Source: three-view drawing plus pictorial views. Frame: mm from the lowest corner of the part. A direction names the side the tool comes from. Give positions to 0.01 mm unless a question says otherwise; leave off trailing zeros. Loops run counter-clockwise (first coordinate to the right, second up) from the corner with the lowest first, then second, coordinate; pieces in that order, holes last. Notation, with made-up numbers: M 46.5,19 L 52.5,19 A18 ccw 52.5,47 Z; hole C 40,39.25 d10. An arc over 180 degrees is marked long. Put each result on its own line as item: value. Start each with the question number.
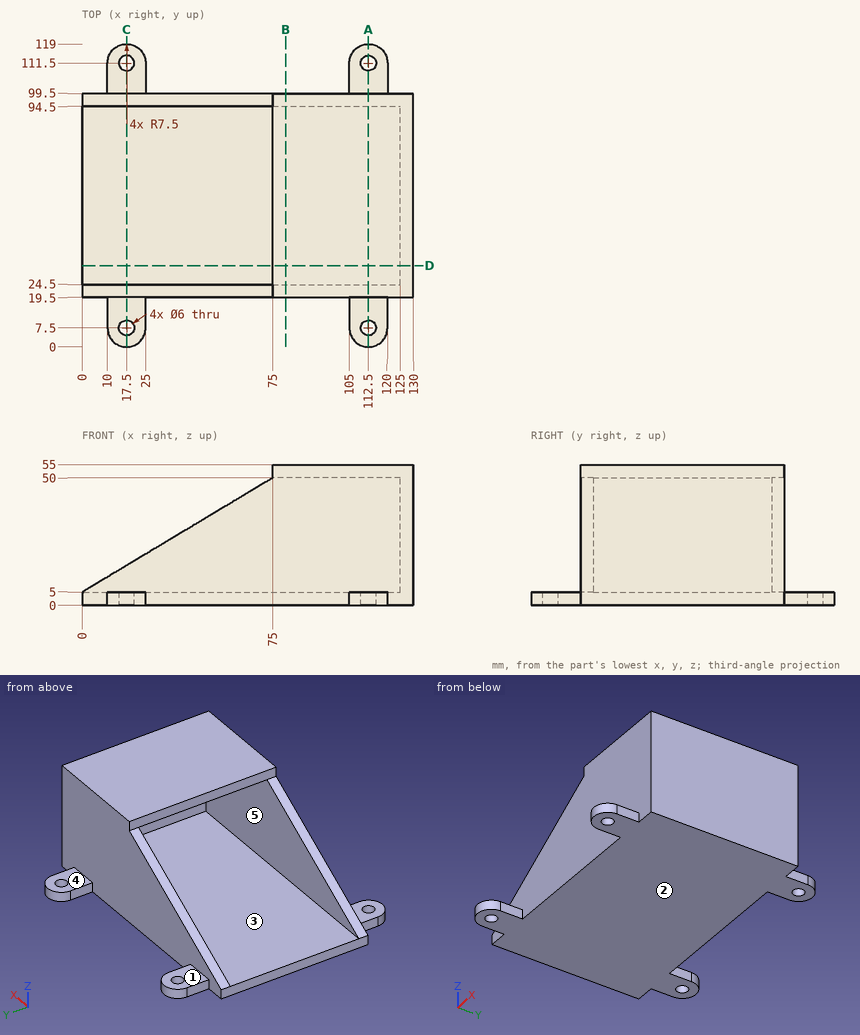
1. Section D-D, the plane y = 32. Output: boundary loops of the cut face in (x, z), plus the area to 3 significant figures.
2. Section A-A, the plane x = 112.5. Output: boundary loops of the cut face in (y, z), plus the area to 4 significant figures.
3. Section C-C, the plane x = 17.5. Output: boundary loops of the cut face in (y, z).
4. Ray query, line 1 (X direction, y = 7.5, z = 1.6); line 2 (Y direction, x = 22, z = 5.5); line 3 (Y direction, x = 112.5, z = 2.6). Return the intervals inside material, ascending.
5. Section B-B, the plane x = 80. Output: boundary loops of the cut face in (y, z), plus the area to 3 significant figures.
6. Set-up query: the marked faces 1, 2 and 3. Return all of +Z, -Z, +X, -X, +Y, -Y with unobstructed straight access to the full face (end or side cutting, diameter ignored); none if empty.
7. Contact query for flat-ended pins moving along their axis: pin 1 (16.5 mm diameter, centred on x = 56, z = 20.5, fed in from -Y); pin 2 (13.5 mm diameter, centred on x = 42, z = 22.5, fed in from +Y); pin 3 (7.5 mm diameter, centred on x = 110, y = 109.5, fed in from +Z). Output: stop coordinate, or through.
8. Pull-direction query (Y, two-part tool) for the marked faces 4 and 5; classes: released by +Y, released by -Y, zero draft, split by the parting line, or undercut.
Results found:
1. outline: M 0,0 L 130,0 L 130,55 L 75,55 L 75,50 L 125,50 L 125,5 L 0,5 Z
1. area: 1,150 mm²
2. outline: M 0,0 L 4.5,0 L 4.5,5 L 0,5 Z; M 10.5,0 L 108.5,0 L 108.5,5 L 99.5,5 L 99.5,55 L 19.5,55 L 19.5,5 L 10.5,5 Z; M 114.5,0 L 119,0 L 119,5 L 114.5,5 Z; hole M 24.5,5 L 94.5,5 L 94.5,50 L 24.5,50 Z
2. area: 1,385 mm²
3. outline: M 0,0 L 4.5,0 L 4.5,5 L 0,5 Z; M 10.5,0 L 108.5,0 L 108.5,5 L 99.5,5 L 99.5,15.5 L 94.5,15.5 L 94.5,5 L 24.5,5 L 24.5,15.5 L 19.5,15.5 L 19.5,5 L 10.5,5 Z; M 114.5,0 L 119,0 L 119,5 L 114.5,5 Z
4. line 1: 10 to 14.5, 20.5 to 25, 105 to 109.5, 115.5 to 120
4. line 2: 19.5 to 24.5, 94.5 to 99.5
4. line 3: 0 to 4.5, 10.5 to 108.5, 114.5 to 119
5. outline: M 19.5,0 L 99.5,0 L 99.5,55 L 19.5,55 Z; hole M 24.5,5 L 94.5,5 L 94.5,50 L 24.5,50 Z
5. area: 1,250 mm²
6. face 1: +Z, +X, -X, +Y
6. face 2: -Z, +X, -X, +Y, -Y
6. face 3: -X
7. pin 1: y = 19.5
7. pin 2: y = 99.5
7. pin 3: z = 5
8. face 4: zero draft
8. face 5: undercut
